Here's how the part is built. I have some questions about the finished solid (model axes, mm). A direction names the side the tool comes from. Round coordinates to 2 decimals unless told otherwise and drop trailing zeros. Order: outer loops, then holes, each group sorted by start corner. A loop starts at its lowest first (then second) coordinate and runs counter-clockwise, first axis right, second up.
```python
from build123d import *

# Parameters (mm, degrees)
SKETCH1_W           = 75
SKETCH1_H           = 50
BOSS_EXTRUDE1_DEPTH = 57
SKETCH2_W           = 22
SKETCH2_H           = 41
CUT_EXTRUDE1_DEPTH  = 46
SKETCH4_W           = 22
SKETCH4_H           = 4
CUT_EXTRUDE2_DEPTH  = 65.399145957
SKETCH5_W           = 4
SKETCH5_H           = 22.4
CUT_EXTRUDE3_DEPTH  = 6
SKETCH6_W           = 1
SKETCH6_H           = 1.5
CUT_EXTRUDE4_DEPTH  = 4.5


with BuildPart() as part:
    # Sketch1 → Boss-Extrude1 (new body)
    with BuildSketch(Plane.XY):
        Rectangle(SKETCH1_W, SKETCH1_H)
    extrude(amount=BOSS_EXTRUDE1_DEPTH)

    # Sketch2 → Cut-Extrude1 (cut)
    with BuildSketch(Plane.XY.offset(57)):
        with Locations((0, 4.5)):
            Rectangle(SKETCH2_W, SKETCH2_H)
    extrude(amount=-CUT_EXTRUDE1_DEPTH, mode=Mode.SUBTRACT)

    # Sketch4 → Cut-Extrude2 (cut, through all)
    with BuildSketch(Plane.XY.offset(11)):
        with Locations((0, 13.8)):
            Rectangle(SKETCH4_W, SKETCH4_H)
    extrude(amount=-CUT_EXTRUDE2_DEPTH, mode=Mode.SUBTRACT)

    # Sketch5 → Cut-Extrude3 (cut)
    with BuildSketch(Plane(origin=(0, 0, 0), x_dir=(-1, 0, 0), z_dir=(0, 0, -1))):
        with Locations((-6, 13.8)):
            Rectangle(SKETCH5_W, SKETCH5_H)
        with Locations((6, 13.8)):
            Rectangle(SKETCH5_W, SKETCH5_H)
    extrude(amount=-CUT_EXTRUDE3_DEPTH, mode=Mode.SUBTRACT)

    # Sketch6 → Cut-Extrude4 (cut)
    with BuildSketch(Plane.XY.offset(11)):
        with Locations((0, 16.55)):
            Rectangle(SKETCH6_W, SKETCH6_H)
    extrude(amount=-CUT_EXTRUDE4_DEPTH, mode=Mode.SUBTRACT)


solid = part.part
```
1. If we section it at D-D, the plane z = 31: Write out the boundary of the cut face in (x, y), and give its area (3 significant figures).
Evaluation:
outline: (-37.5, -25) - (37.5, -25) - (37.5, 25) - (11, 25) - (11, -16) - (-11, -16) - (-11, 25) - (-37.5, 25) - close
area: 2,850 mm2
2. If we section it at B-B, the plane z = 10: Write out the boundary of the cut face in (x, y), and give its area (3 significant figures).
Evaluation:
outline: (-37.5, -25) - (37.5, -25) - (37.5, 25) - (-37.5, 25) - close; hole (-11, 11.8) - (11, 11.8) - (11, 15.8) - (0.5, 15.8) - (0.5, 17.3) - (-0.5, 17.3) - (-0.5, 15.8) - (-11, 15.8) - close
area: 3,660 mm2
3. If we section it at C-C, the plane y = -12: Write out the boundary of the cut face in (x, z).
Evaluation:
outline: (-37.5, 0) - (37.5, 0) - (37.5, 57) - (11, 57) - (11, 11) - (-11, 11) - (-11, 57) - (-37.5, 57) - close
4. If we mould it in two halves opening along X, with no side actions, what happens to faces 4 (the flat face through (-1, 0, 0)), 5 (the flat face through (0, 15.8, 6)), 6 (the flat face through (37.5, 0, 28))? For each: released by +X, released by -X, zero draft, split by the parting line, or undercut.
Evaluation:
face 4: zero draft
face 5: undercut
face 6: released by +X
5. I need wall thicknesses on probe 1 along X at (y, z) = (11.5, 13); probe 2 along Y at (x, z) = (1, 28); probe 3 along Z at (x, y) = (2.5, 1). Which ranges of each line are inside material? Lowest first, please.
Evaluation:
probe 1: x = -37.5 to -11, 11 to 37.5
probe 2: y = -25 to -16
probe 3: z = 0 to 11
6. If we section it at A-A, the plane x = -5.5: Write out the boundary of the cut face in (y, z).
Evaluation:
outline: (-25, 0) - (2.6, 0) - (2.6, 6) - (11.8, 6) - (11.8, 11) - (-16, 11) - (-16, 57) - (-25, 57) - close; (15.8, 6) - (25, 6) - (25, 11) - (15.8, 11) - close
7. On a 3-axis mill with a long thin cutter (end or side, diameter ignored), from which of +Z, -Z, +X, -X, +Y, -Y can I reach the whole of each face in a straight line? I mean faces 1 (the flat face through (0, -2, 11)), 2 (the flat face through (-37.5, 0, 28)), 3 (the flat face through (6, 2.6, 3)). Say none if no direction works.
Evaluation:
face 1: +Z, +Y
face 2: +Z, -Z, -X, +Y, -Y
face 3: -Z, +Y
8. I'm going to push flat-ended pins straight in: P1, Ø11, axis at x = 2, y = -0.5, coming from the +Z side; P2, Ø17.5, axis at x = -2, z = 30, coming from the +Y side; P3, Ø1.2, axis at x = -6.5, z = 2, coming from the +Y side. Where does each tip first touch, or does it pass through?
Evaluation:
P1: stops at z = 11
P2: stops at y = -16
P3: stops at y = 2.6
